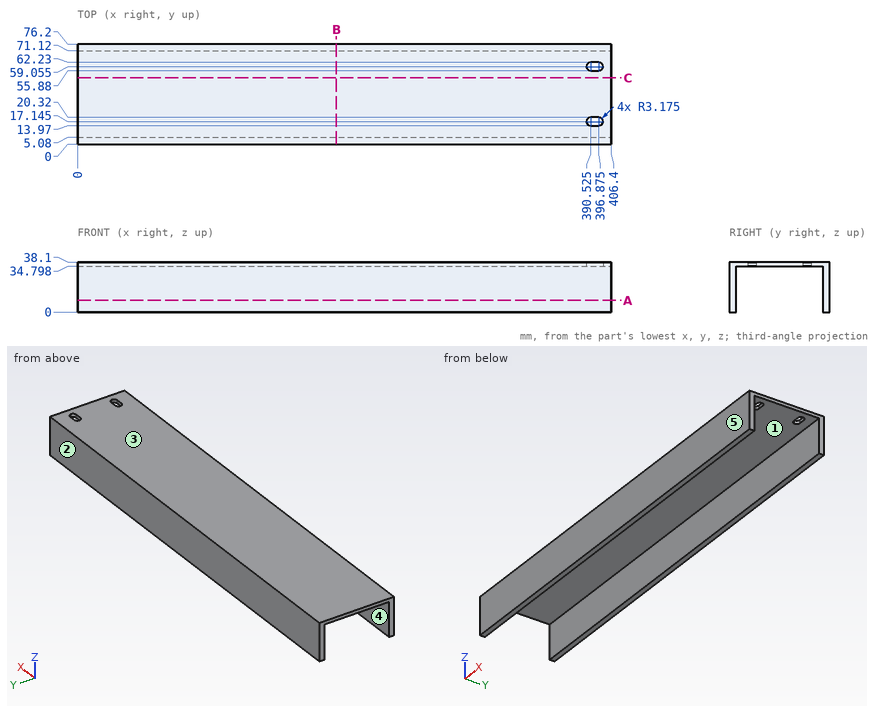
Here's the drawing with two shaded views (mm, measured from the low corner). I have some questions. A direction names the side the tool comes from. Coordinates: 2 decimals unless noted, no trailing zeros. Write each loop counter-clockwise with the first axis right and the second up, starting at its lowest first coordinate (ties: lowest second). Pieces come first, ordered by that corner, then holes. Notation, with made-up numbers: (54.25, -28.75) -> (107.25, -28.75) arc R24 cw to (107.25, -0.75) -> close; hole circle Ø5 at (39, 17). An arc over 180 degrees is marked (long way). Use a Markdown table: item, result. Add a question column.
(1) If we section it at A-A, the plane z = 9: Write out the boundary of the cut face in (x, y), and give its area (3 significant figures).
(2) Please list where these lines run through material, in increasing order: line 1 (Y direction, x = 349.5, z = 14); line 2 (Z direction, x = 198, y = 8).
(3) If we section it at C-C, the plane y = 50.5: Write out the boundary of the cut face in (x, z), and give its area (3 significant figures).
(4) We'd pull the mould along Y, two halves only. Please class the marked faces 1, 2 and 3: +Y half, -Y half, draft (parallel to the pull), parting line (faces both ways), or undercut.
(5) If we section it at B-B, the plane x = 197: Write out the boundary of the cut face in (y, z).
(6) For the marked faces 4 and 5, which set-ups out of +Z, -Z, +X, -X, +Y, -Y let a thin tool reach every point of the face, with its end or its side?
(7) I'm going to push a flat-ended pin straight in: P1, Ø4, axis at x = 359.5, y = 34.5, coming from the -Z side. Where does the tip first touch, or does it pass through?
Outcome:
| question | item | result |
|---|---|---|
| 1 | outline | (0, 0) -> (406.4, 0) -> (406.4, 5.08) -> (0, 5.08) -> close; (0, 71.12) -> (406.4, 71.12) -> (406.4, 76.2) -> (0, 76.2) -> close |
| 1 | area | 4,130 mm^2 |
| 2 | line 1 | y = 0 to 5.08, 71.12 to 76.2 |
| 2 | line 2 | z = 34.8 to 38.1 |
| 3 | outline | (0, 34.8) -> (406.4, 34.8) -> (406.4, 38.1) -> (0, 38.1) -> close |
| 3 | area | 1,340 mm^2 |
| 4 | face 1 | undercut |
| 4 | face 2 | +Y half |
| 4 | face 3 | draft |
| 5 | outline | (0, 0) -> (5.08, 0) -> (5.08, 34.8) -> (71.12, 34.8) -> (71.12, 0) -> (76.2, 0) -> (76.2, 38.1) -> (0, 38.1) -> close |
| 6 | face 4 | -Z, +X, -X |
| 6 | face 5 | +Z, -Z, +X, -X, -Y |
| 7 | P1 | stops at z = 34.8 |
